```python
from build123d import *

# Parameters (mm, degrees)
SKETCH1_W           = 90
SKETCH1_H           = 90
BOSS_EXTRUDE1_DEPTH = 160
SKETCH2_W           = 2.27948718
SKETCH2_H           = 9.280769231
SKETCH2_W_2         = 2.279487179
SKETCH2_H_2         = 13.025641026
CUT_EXTRUDE1_DEPTH  = 150


with BuildPart() as part:
    # Sketch1 → Boss-Extrude1 (new body)
    with BuildSketch(Plane(origin=(0, 0, 0), x_dir=(1, 0, 0), z_dir=(0, 1, 0))):
        with Locations((45, 45)):
            Rectangle(SKETCH1_W, SKETCH1_H)
    extrude(amount=BOSS_EXTRUDE1_DEPTH)

    # Sketch2 → Cut-Extrude1 (cut)
    with BuildSketch(Plane(origin=(0, 160, 0), x_dir=(1, 0, 0), z_dir=(0, 1, 0))):
        with BuildLine():
            Line((21.611077672, 65.922158503), (24.483333281, 65.922158503))
            add(Edge.make_bspline(
                [(24.483333281, 65.922158503), (24.707258642, 65.920593189), (25.140108898, 65.917567417), (25.767223285, 65.88347425), (26.350359864, 65.831041379), (26.889894536, 65.758910462), (27.384721167, 65.663461507), (27.834201687, 65.543739501), (28.239844663, 65.405540361), (28.606097885, 65.242921031), (28.940451848, 65.053323041), (29.257931608, 64.842126103), (29.557913799, 64.601593454), (29.844608198, 64.336365449), (30.114314952, 64.041589823), (30.371525645, 63.722149129), (30.609942592, 63.373411035), (30.836772622, 63.003737182), (31.0419102, 62.611560926), (31.220838862, 62.200220391), (31.370728486, 61.772362706), (31.492521568, 61.327531886), (31.589604711, 60.867204634), (31.657531829, 60.390452053), (31.69952505, 59.897715535), (31.703784912, 59.563763804), (31.705949466, 59.394073568)],
                knots=[0, 0, 0, 0, 1.44355588, 2.790409838, 4.047694926, 5.217575253, 6.298404546, 7.294384826, 8.214239204, 9.058592145, 9.873746385, 10.689560431, 11.514393297, 12.350027578, 13.205127629, 14.088021785, 14.991911688, 15.926770944, 16.882954281, 17.842803888, 18.816321264, 19.80318086, 20.814351908, 21.847355356, 22.906180909, 24, 24, 24, 24], degree=3))
            add(Edge.make_bspline(
                [(31.705949466, 59.394073568), (31.700281493, 59.154629598), (31.689123756, 58.683270128), (31.595137212, 57.991555537), (31.443129146, 57.328478111), (31.229391999, 56.699224698), (30.964415152, 56.109398894), (30.647870638, 55.569402028), (30.284399734, 55.082132531), (29.8782369, 54.650016606), (29.438461471, 54.278607111), (28.981446119, 53.960522058), (28.502738681, 53.709685452), (28.080930527, 53.550617534), (27.715170235, 53.451691051), (27.394036655, 53.393224547), (27.029261674, 53.339607236), (26.617444083, 53.298172932), (26.160390436, 53.261223715), (25.656278912, 53.241146949), (25.106741679, 53.224466136), (24.725036111, 53.22294787), (24.526582479, 53.222158503)],
                knots=[0, 0, 0, 0, 1.315458931, 2.589557908, 3.828601765, 5.048913369, 6.235739168, 7.376350998, 8.481830359, 9.569842114, 10.627874879, 11.640079404, 12.624025415, 13.590060155, 14.111227486, 14.704434459, 15.382649715, 16.137166398, 16.978595427, 17.902333227, 18.909396075, 20, 20, 20, 20], degree=3))
            Line((24.526582479, 53.222158503), (21.611077672, 53.222158503))
            Line((21.611077672, 53.222158503), (21.611077672, 65.922158503))
        make_face()
        with BuildLine():
            Line((23.890564851, 63.642671324), (23.890564851, 55.501645683))
            Line((23.890564851, 55.501645683), (25.081189851, 55.501645683))
            add(Edge.make_bspline(
                [(25.081189851, 55.501645683), (25.222855941, 55.501905274), (25.495326993, 55.502404554), (25.888713514, 55.52618568), (26.252496301, 55.550055373), (26.585673943, 55.595360849), (26.890671205, 55.645827961), (27.163298221, 55.716059857), (27.409175021, 55.789832515), (27.625298266, 55.883754252), (27.823249549, 55.989469418), (28.006529826, 56.11332699), (28.183446608, 56.250866153), (28.350692293, 56.406132129), (28.508899865, 56.577068904), (28.657133269, 56.764557241), (28.797371028, 56.968025107), (28.926013504, 57.188548286), (29.043567688, 57.423798005), (29.147851421, 57.671495526), (29.234318024, 57.933703637), (29.306183771, 58.207967754), (29.357539996, 58.496675658), (29.400027477, 58.797688929), (29.421931011, 59.112200156), (29.424937135, 59.326204107), (29.426462287, 59.434778696)],
                knots=[0, 0, 0, 0, 1.50275155, 2.890291501, 4.180787663, 5.369391935, 6.45668281, 7.458360028, 8.354766181, 9.177074746, 9.954075863, 10.732690366, 11.5210699, 12.329727389, 13.151100085, 13.990027547, 14.863562427, 15.770965086, 16.696477834, 17.652329173, 18.619756807, 19.62365428, 20.657822005, 21.729286259, 22.847956731, 24, 24, 24, 24], degree=3))
            add(Edge.make_bspline(
                [(29.426462287, 59.434778696), (29.423424701, 59.601158989), (29.417501644, 59.92558767), (29.360380967, 60.398125124), (29.267399399, 60.843089927), (29.134723662, 61.258830694), (28.967481782, 61.646515876), (28.758139585, 62.002860957), (28.515706351, 62.333852044), (28.323996765, 62.528022037), (28.228205075, 62.625043119)],
                knots=[0, 0, 0, 0, 1.13821349, 2.219428113, 3.251817212, 4.244760574, 5.201143372, 6.134805572, 7.068016741, 8, 8, 8, 8], degree=3))
            add(Edge.make_bspline(
                [(28.228205075, 62.625043119), (28.133745399, 62.707718197), (27.940822207, 62.876572683), (27.602112479, 63.078903538), (27.228871901, 63.256671027), (26.812561848, 63.39762082), (26.357205771, 63.509089926), (25.86009156, 63.585967442), (25.32388137, 63.635368119), (24.952407444, 63.640184767), (24.760636966, 63.642671324)],
                knots=[0, 0, 0, 0, 0.813307809, 1.661089106, 2.549956539, 3.493439533, 4.508053171, 5.589449661, 6.755572447, 8, 8, 8, 8], degree=3))
            Line((24.760636966, 63.642671324), (23.890564851, 63.642671324))
        make_face(mode=Mode.SUBTRACT)
        with BuildLine():
            Line((33.334154595, 62.502927734), (35.288000749, 62.502927734))
            Line((35.288000749, 62.502927734), (35.288000749, 61.360640074))
            add(Edge.make_bspline(
                [(35.288000749, 61.360640074), (35.343271305, 61.462155493), (35.451299902, 61.66057159), (35.649757493, 61.926905908), (35.877753612, 62.151205239), (36.127095654, 62.338161009), (36.398539324, 62.483874674), (36.684815845, 62.587714031), (36.983476127, 62.655195223), (37.187212046, 62.662205243), (37.290184242, 62.665748247)],
                knots=[0, 0, 0, 0, 1.09866127, 2.147379032, 3.14564304, 4.131443017, 5.102343063, 6.064490016, 7.021754664, 8, 8, 8, 8], degree=3))
            add(Edge.make_bspline(
                [(37.290184242, 62.665748247), (37.364954905, 62.662247019), (37.517214674, 62.655117269), (37.749279987, 62.613671922), (37.984693596, 62.538730853), (38.139616036, 62.471256381), (38.218769979, 62.436781901)],
                knots=[0, 0, 0, 0, 0.931404136, 1.896671404, 2.925354185, 4, 4, 4, 4], degree=3))
            Line((38.218769979, 62.436781901), (37.511518377, 60.505832382))
            add(Edge.make_bspline(
                [(37.511518377, 60.505832382), (37.448300183, 60.536376356), (37.329474315, 60.593787271), (37.156959787, 60.661538064), (37.000395699, 60.702876287), (36.901136942, 60.709044312), (36.855148184, 60.711902093)],
                knots=[0, 0, 0, 0, 1.214386998, 2.282580073, 3.20428172, 4, 4, 4, 4], degree=3))
            add(Edge.make_bspline(
                [(36.855148184, 60.711902093), (36.811725854, 60.710008376), (36.726306649, 60.706283109), (36.600230293, 60.674358835), (36.481492619, 60.619306412), (36.364371666, 60.548778795), (36.258106978, 60.450740133), (36.151907928, 60.337242974), (36.058319638, 60.197115636), (35.959556851, 60.041146791), (35.875463869, 59.850241066), (35.803356726, 59.622338971), (35.739108683, 59.354803523), (35.694897257, 59.046214239), (35.65216514, 58.699557253), (35.626729934, 58.312288146), (35.607772753, 57.8856315), (35.606613649, 57.587809763), (35.606009563, 57.432595202)],
                knots=[0, 0, 0, 0, 0.544232178, 1.070598461, 1.618251235, 2.182094276, 2.777567932, 3.425210017, 4.127676488, 4.886675562, 5.738955394, 6.734782583, 7.883056018, 9.186093582, 10.642914445, 12.264202625, 14.053029461, 16, 16, 16, 16], degree=3))
            Line((35.606009563, 57.432595202), (35.613641774, 56.979750651))
            Line((35.613641774, 56.979750651), (35.613641774, 53.222158503))
            Line((35.613641774, 53.222158503), (33.334154595, 53.222158503))
            Line((33.334154595, 53.222158503), (33.334154595, 62.502927734))
        make_face()
        with BuildLine():
            add(Edge.make_bspline(
                [(40.330348505, 66.410620042), (40.428594386, 66.405799727), (40.62150964, 66.396334575), (40.897886993, 66.304070393), (41.151545391, 66.159264517), (41.375786449, 65.960587403), (41.562289193, 65.723330591), (41.704784215, 65.457705815), (41.784162256, 65.163402119), (41.795186692, 64.960100203), (41.800821261, 64.856192959)],
                knots=[0, 0, 0, 0, 0.989868614, 1.943702388, 2.910836514, 3.924849579, 4.949916355, 5.946401046, 6.950409252, 8, 8, 8, 8], degree=3))
            add(Edge.make_bspline(
                [(41.800821261, 64.856192959), (41.795388287, 64.753051453), (41.784801879, 64.552075317), (41.702957281, 64.261766931), (41.566181513, 63.996271169), (41.378168214, 63.762538061), (41.156358222, 63.56706076), (40.908242454, 63.41962602), (40.634513598, 63.332494474), (40.444591807, 63.322238088), (40.348156999, 63.317030298)],
                knots=[0, 0, 0, 0, 1.05296456, 2.051751585, 3.055639087, 4.085634717, 5.099016424, 6.062201612, 7.016062274, 8, 8, 8, 8], degree=3))
            add(Edge.make_bspline(
                [(40.348156999, 63.317030298), (40.249053512, 63.321833381), (40.054459903, 63.331264425), (39.775815687, 63.423744483), (39.518774135, 63.567409919), (39.295505833, 63.770146314), (39.106867216, 64.009089016), (38.970596432, 64.280897766), (38.885355686, 64.577213904), (38.875237684, 64.783526859), (38.870052031, 64.889265875)],
                knots=[0, 0, 0, 0, 0.989065327, 1.942068821, 2.907541208, 3.917690034, 4.939857478, 5.938239964, 6.943311734, 8, 8, 8, 8], degree=3))
            add(Edge.make_bspline(
                [(38.870052031, 64.889265875), (38.87569544, 64.990655977), (38.886781102, 65.189822194), (38.966634626, 65.477582657), (39.105862243, 65.738741864), (39.291021589, 65.971655469), (39.513293056, 66.166626507), (39.766799179, 66.307034534), (40.041316502, 66.395487942), (40.233009707, 66.405523927), (40.330348505, 66.410620042)],
                knots=[0, 0, 0, 0, 1.038616768, 2.040212704, 3.031499824, 4.052181184, 5.074969369, 6.039807101, 7.004644834, 8, 8, 8, 8], degree=3))
        make_face()
        with Locations((40.335436646, 57.862543118)):
            Rectangle(SKETCH2_W, SKETCH2_H)
        with Locations((44.56876998, 59.734979016)):
            Rectangle(SKETCH2_W_2, SKETCH2_H_2)
        with Locations((48.802103313, 59.734979016)):
            Rectangle(SKETCH2_W_2, SKETCH2_H_2)
    extrude(amount=-CUT_EXTRUDE1_DEPTH, mode=Mode.SUBTRACT)


solid = part.part
```
CAD build for the part. Positions are in the model's coordinates, mm. A direction names the side the tool comes from. Coordinates: 2 decimals unless noted, no trailing zeros. Write each question's results on one line, items separated by ' | '. Start each with the question number.
Q1. Cut at A-A (y = 14.5). Count the separate pieces of the cut face and the enclosed holes in it, then the cut area to 3 significant figures.
Q2. Which spindle directions (+Z, -Z, +X, -X, +Y, -Y) get a long thin tool onto all of the face, cutting with end or side? Do faces 4 (the flat face through (44, 0, -46)), 5 (the flat face through (35, 10, -59)). Say none if no direction does.
Q3. Pull direction X, two halves, no side cores. Call faces 1 (the flat face through (27, 160, -60)), 2 (the flat face through (45.709, 86, -60)), 3 (the flat face through (0, 79, -44)): +X half, -X half, draft (parallel to the pull), parting line (faces both ways), or undercut.
Q4. Drill centre lines: probe 1 along Z at (x, y) = (29, 78.5); probe 2 along Z at (x, y) = (26.5, 120.5); probe 3 along Z at (x, y) = (23.5, 54.5). Where is each one in solid material? Low to high. Write a range as from..to.
Found:
1) separate pieces: 2 | enclosed holes: 6 | area: 7,910 mm²
2) face 4: +Z, -Z, +X, -X, -Y | face 5: +Y
3) face 1: draft | face 2: undercut | face 3: -X half
4) probe 1: -90..-65.01, -61.56..-57.34, -53.99..0 | probe 2: -90..-65.81, -63.47..-55.58, -53.29..0 | probe 3: -90..-65.92, -53.22..0
